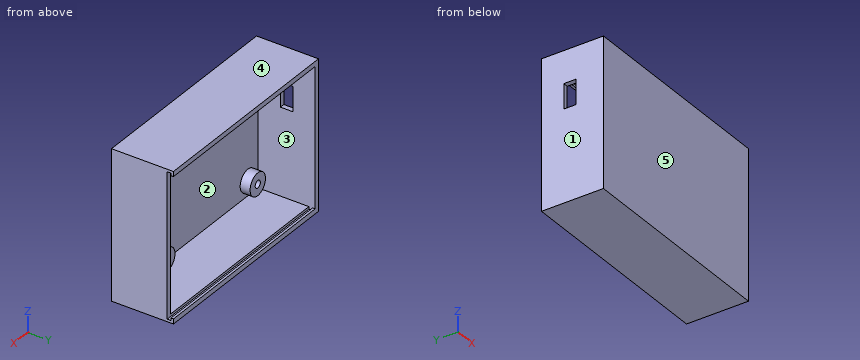
```python
from build123d import *

# Parameters (mm, degrees)
SKIZZE1_W                       = 85
SKIZZE1_H                       = 60
AUFSATZ_LINEAR_AUSTRAGEN1_DEPTH = 25
WANDUNG1_T                      = -2
SKIZZE2_R                       = 4.5
SKIZZE2_R_2                     = 1.5
AUFSATZ_LINEAR_AUSTRAGEN2_DEPTH = 4
SCHNITT_LINEAR_AUSTRAGEN1_REACH = 87
SKIZZE3_W                       = 10
SKIZZE3_H                       = 5
SCHNITT_LINEAR_AUSTRAGEN2_REACH = 87
SKIZZE4_W                       = 56
SKIZZE4_H                       = 1
SKIZZE5_W                       = 58
SKIZZE5_H                       = 1.5
SCHNITT_LINEAR_AUSTRAGEN3_DEPTH = 83


with BuildPart() as part:
    # Skizze1 → Aufsatz-Linear austragen1 (new body)
    with BuildSketch(Plane(origin=(0, 0, 0), x_dir=(1, 0, 0), z_dir=(0, 1, 0))):
        with Locations((42.5, 30)):
            Rectangle(SKIZZE1_W, SKIZZE1_H)
    extrude(amount=AUFSATZ_LINEAR_AUSTRAGEN1_DEPTH)

    # Wandung1
    wandung1_openings = [part.faces().sort_by_distance(p)[0] for p in [
        (42.5, 25, -30),
    ]]
    offset(amount=WANDUNG1_T, openings=wandung1_openings, kind=Kind.INTERSECTION)

    # Skizze2 → Aufsatz-Linear austragen2 (add)
    with BuildSketch(Plane(origin=(0, 2, 0), x_dir=(1, 0, 0), z_dir=(0, 1, 0))):
        with Locations((8, 52)):
            Circle(SKIZZE2_R)
        with Locations((8, 52)):
            Circle(SKIZZE2_R_2, mode=Mode.SUBTRACT)
        with Locations((61, 54)):
            Circle(SKIZZE2_R)
        with Locations((61, 54)):
            Circle(SKIZZE2_R_2, mode=Mode.SUBTRACT)
        with Locations((68, 13)):
            Circle(SKIZZE2_R)
        with Locations((68, 13)):
            Circle(SKIZZE2_R_2, mode=Mode.SUBTRACT)
    extrude(amount=AUFSATZ_LINEAR_AUSTRAGEN2_DEPTH)

    # Skizze3 → Schnitt-Linear austragen1 (cut, up to next)
    with BuildSketch(Plane.ZY, mode=Mode.PRIVATE) as schnitt_linear_austragen1_sk1:
        with Locations((-18, 13.5)):
            Rectangle(SKIZZE3_W, SKIZZE3_H)
    schnitt_linear_austragen1_tool1 = extrude(schnitt_linear_austragen1_sk1.sketch, amount=-SCHNITT_LINEAR_AUSTRAGEN1_REACH, mode=Mode.PRIVATE) & part.part
    add(schnitt_linear_austragen1_tool1.solids().sort_by_distance((0, 13.5, -18))[0], mode=Mode.SUBTRACT)

    # Skizze4 → Schnitt-Linear austragen2 (cut, up to next)
    with BuildSketch(Plane(origin=(85, 0, 0), x_dir=(0, 0, -1), z_dir=(1, 0, 0)), mode=Mode.PRIVATE) as schnitt_linear_austragen2_sk1:
        with Locations((30, 24.5)):
            Rectangle(SKIZZE4_W, SKIZZE4_H)
    schnitt_linear_austragen2_tool1 = extrude(schnitt_linear_austragen2_sk1.sketch, amount=-SCHNITT_LINEAR_AUSTRAGEN2_REACH, mode=Mode.PRIVATE) & part.part
    add(schnitt_linear_austragen2_tool1.solids().sort_by_distance((85, 24.5, -30))[0], mode=Mode.SUBTRACT)

    # Skizze5 → Schnitt-Linear austragen3 (cut)
    with BuildSketch(Plane(origin=(85, 0, 0), x_dir=(0, 0, -1), z_dir=(1, 0, 0))):
        with Locations((30, 23.25)):
            Rectangle(SKIZZE5_W, SKIZZE5_H)
    extrude(amount=-SCHNITT_LINEAR_AUSTRAGEN3_DEPTH, mode=Mode.SUBTRACT)


solid = part.part
```
Can you work these out from the model? Positions are in its coordinate system, mm. Face numbers are marked on the shaded views. A direction names the side the tool comes from. Coordinates: 2 decimals unless noted, no trailing zeros. Order: outer loops, then holes, each group sorted by start corner. A loop starts at its lowest first (then second) coordinate and runs counter-clockwise, first axis right, second up. Notation, with made-up numbers: (76.5, 45) - (115.5, 45) arc R4 ccw to (115.5, 52) - close; hole circle Ø1 at (47, 59.5). An arc over 180 degrees is marked (long way). Answer in a Markdown table with one row per item.
1. Suppose I cut it at D-D (y = 13). Please give me the cut outline in (x, z).
Reply:
| item | result |
|---|---|
| outline | (0, -60) - (85, -60) - (85, 0) - (0, 0) - (0, -13) - (2, -13) - (2, -2) - (83, -2) - (83, -58) - (2, -58) - (2, -23) - (0, -23) - close |
2. If we mould it in two halves opening along Z, with no side actions, what happens to the marked faces 3, 4 and 5? For each: pulls with the +Z half, pulls with the -Z half, needs draft (parallel to the pull), parting line crosses it, or undercut.
Reply:
| item | result |
|---|---|
| face 3 | undercut |
| face 4 | pulls with the +Z half |
| face 5 | needs draft |
3. Suppose I cut it at C-C (z = -7). Please give me the cut outline in (x, y), and give its area (3 significant figures).
Reply:
| item | result |
|---|---|
| outline | (0, 0) - (85, 0) - (85, 22.5) - (83, 22.5) - (83, 2) - (2, 2) - (2, 25) - (0, 25) - close |
| area | 257 mm^2 |
4. For pin 1 (5 mm diameter, centred on x = 68, z = -13, fed in from +Y); pin 2 (1.5 mm diameter, centred on x = 68.5, z = -13.5, fed in from +Y), each with a flat end and sliding along its axis, tell me the tip position at first contact or that it passes through.
Reply:
| item | result |
|---|---|
| pin 1 | stops at y = 6 |
| pin 2 | stops at y = 2 |
5. Suppose I cut it at A-A (y = 18.5). Please give me the cut outline in (x, z), and give its area (3 significant figures).
Reply:
| item | result |
|---|---|
| outline | (0, -60) - (85, -60) - (85, 0) - (0, 0) - close; hole (2, -58) - (83, -58) - (83, -2) - (2, -2) - close |
| area | 564 mm^2 |
6. Suppose I cut it at B-B (x = 61). Please give me the cut outline in (y, z).
Reply:
| item | result |
|---|---|
| outline | (0, -60) - (25, -60) - (25, -58) - (24, -58) - (24, -59) - (22.5, -59) - (22.5, -58) - (6, -58) - (6, -55.5) - (2, -55.5) - (2, -52.5) - (6, -52.5) - (6, -49.5) - (2, -49.5) - (2, -2) - (22.5, -2) - (22.5, -1) - (24, -1) - (24, -2) - (25, -2) - (25, 0) - (0, 0) - close |
7. If I drill on line 1 along Z through (x, y) = (61, 5.05); line 2 along Z through (x, y) = (68, 4.65); line 3 along Z through (x, y) = (49, 23.25), over which ranges is the centre line in solid material (lowest first)?
Reply:
| item | result |
|---|---|
| line 1 | z = -60 to -55.5, -52.5 to -49.5, -2 to 0 |
| line 2 | z = -60 to -58, -17.5 to -14.5, -11.5 to -8.5, -2 to 0 |
| line 3 | z = -60 to -59, -1 to 0 |
8. For the marked faces 1 and 2, which set-ups out of +Z, -Z, +X, -X, +Y, -Y let a thin tool reach every point of the face, with its end or its side?
Reply:
| item | result |
|---|---|
| face 1 | +Z, -Z, -X, +Y, -Y |
| face 2 | +Y |
